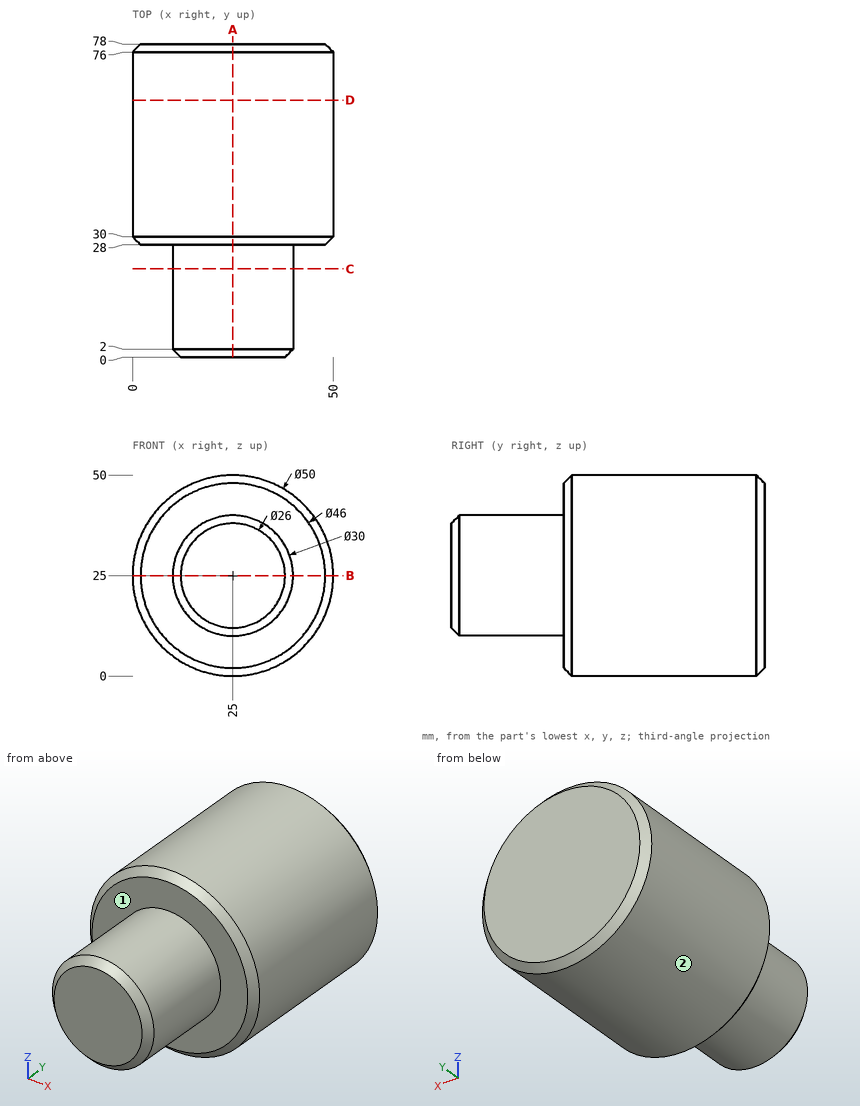
Part print with two shaded views. Sizes in mm from the minimum x, y, z corner. A direction names the side the tool comes from. Round coordinates to 2 decimals unless told otherwise and drop trailing zeros. Order: outer loops, then holes, each group sorted by start corner. A loop starts at its lowest first (then second) coordinate and runs counter-clockwise, first axis right, second up. Notation, with made-up numbers: (24, 46) - (45, 46) arc R30 ccw to (45, 78) - close; hole circle Ø2 at (-25, -6.75). An arc over 180 degrees is marked (long way). Answer in a Markdown table with one row per item. Add a question column.
(1) Band-saw the part on D-D on y = 64. List the corners of the cut face in (x, z).
(2) Band-saw the part on B-B on z = 25. List the corners of the cut face in (x, y).
(3) Probe L1, parallel to Y at x = 31.5, z = 39; L2, parallel to Z at x = 5, y = 40.5; L3, parallel to X at y = 40.5, z = 16. List the from-to ranges inside material, lowest first. Write a range as [from, to].
(4) Drop flat-ended pins along their axis: pin 1 Ø8 at (x, y) = (6, 29) entering from +Z; pin 2 Ø1.5 at (x, y) = (25.5, 11) entering from -Z; pin 3 Ø1.5 at (x, y) = (43.5, 66) entering from +Z. Give the stop position or say it passes through.
(5) 3-axis set-ups, long thin cutter, end or side, ignore diameter. For the marked faces 1 and 2: which of +Z, -Z, +X, -X, +Y, -Y reach the whole face in a straight line?
(6) Band-saw the part on C-C on y = 22. List the corners of the cut face in (x, z), and give its area (3 significant figures).
(7) Band-saw the part on A-A on x = 25. List the corners of the cut face in (y, z).
Data:
| question | item | result |
|---|---|---|
| 1 | outline | circle Ø50 at (25, 25) |
| 2 | outline | (0, 30) - (2, 28) - (10, 28) - (10, 2) - (12, 0) - (38, 0) - (40, 2) - (40, 28) - (48, 28) - (50, 30) - (50, 76) - (48, 78) - (2, 78) - (0, 76) - close |
| 3 | L1 | y = [28, 78] |
| 3 | L2 | z = [10, 40] |
| 3 | L3 | x = [1.68, 48.32] |
| 4 | pin 1 | stops at z = 44.9 |
| 4 | pin 2 | stops at z = 10 |
| 4 | pin 3 | stops at z = 42.61 |
| 5 | face 1 | -Y |
| 5 | face 2 | +Y, -Y |
| 6 | outline | circle Ø30 at (25, 25) |
| 6 | area | 707 mm^2 |
| 7 | outline | (0, 12) - (2, 10) - (28, 10) - (28, 2) - (30, 0) - (76, 0) - (78, 2) - (78, 48) - (76, 50) - (30, 50) - (28, 48) - (28, 40) - (2, 40) - (0, 38) - close |
